```python
from build123d import *

# Parameters (mm, degrees)
F1_DEPTH = 63.5
F2_DEPTH = 25.4
F3_DEPTH = 7.9375
F5_R     = 6.35


with BuildPart() as f1:
    # F0 (on Front) → F1 (new body, symmetric)
    with BuildSketch(Plane.XZ):
        Polygon((12.7672983825, 16.0020012408), (-31.8172983825, 16.0020012408), (-31.8172983825, -16.0020012408), (31.8172983825, -16.0020012408), (31.8172983825, 16.0020012408), align=None)
    extrude(amount=F1_DEPTH, both=True)

    # F0 (on Front) → F2 (join, symmetric)
    with BuildSketch(Plane.XZ):
        with BuildLine():
            Line((12.7672983825, 20.5231987592), (12.7672983825, 16.0020012408))
            Line((12.7672983825, 16.0020012408), (31.8172983825, 16.0020012408))
            Line((31.8172983825, 16.0020012408), (31.8172983825, 20.5231987592))
            ThreePointArc((31.8172983825, 20.5231987592), (36.3344606658, 31.6144181421), (47.3152697086, 36.3937209427))
            Line((47.3152697086, 36.3937209427), (47.3152697086, 55.4461636158))
            ThreePointArc((47.3152697086, 55.4461636158), (22.8636521102, 45.0852416156), (12.7672983825, 20.5231987592))
        make_face()
        with BuildLine():
            ThreePointArc((47.6922983825, 55.4481987592), (47.5037812992, 55.4476899696), (47.3152697086, 55.4461636158))
            Line((47.3152697086, 55.4461636158), (47.3152697086, 36.3937209427))
            ThreePointArc((47.3152697086, 36.3937209427), (47.5037707507, 36.3970792656), (47.6922983825, 36.3981987592))
            Line((47.6922983825, 36.3981987592), (76.2672983825, 36.3981987592))
            Line((76.2672983825, 36.3981987592), (76.2672983825, 55.4481987592))
            Line((76.2672983825, 55.4481987592), (47.6922983825, 55.4481987592))
        make_face()
    extrude(amount=F2_DEPTH, both=True)

    # F0 (on Front) → F3 (join, symmetric)
    with BuildSketch(Plane.XZ):
        with BuildLine():
            add(Edge.make_bspline(
                [(47.3152697086, 55.447760652), (14.70907961, 55.3720610373), (-31.8172983825, 45.4738341579), (-31.8172983825, 16.0020012408)],
                knots=[0.3413515557, 0.3413515557, 0.3413515557, 0.3413515557, 88.7568503068, 88.7568503068, 88.7568503068, 88.7568503068], degree=3))
            Line((-31.8172983825, 16.0020012408), (12.7672983825, 16.0020012408))
            Line((12.7672983825, 16.0020012408), (12.7672983825, 20.5231987592))
            ThreePointArc((12.7672983825, 20.5231987592), (22.8636521102, 45.0852416156), (47.3152697086, 55.4461636158))
            Line((47.3152697086, 55.4461636158), (47.3152697086, 55.447760652))
        make_face()
    extrude(amount=F3_DEPTH, both=True)

    # F0 (on Front) → F4 (revolve)
    with BuildSketch(Plane.XZ):
        Polygon((98.1152697086, 60.1979987592), (76.2672983825, 60.1979987592), (76.2672983825, 55.4481987592), (76.2672983825, 36.3981987592), (76.2672983825, 31.6229987592), (98.1152697086, 31.6229987592), align=None)
    revolve(axis=Axis((76.2672983825, 0, 45.9104987592), (0, 0, -1)))

    # F5
    f5_edges = [f1.edges().sort_by_distance(p)[0] for p in [
        (31.817298, -63.5, 0),
        (-31.817298, -63.5, 0),
        (-31.817298, 63.5, 0),
        (31.817298, 63.5, 0),
        (0, -63.5, 16.002001),
        (0, -63.5, -16.002001),
        (31.817298, -44.45, 16.002001),
        (31.817298, 0, -16.002001),
        (-31.817298, 35.71875, 16.002001),
        (-31.817298, -35.71875, 16.002001),
        (-31.817298, 0, -16.002001),
        (0, 63.5, 16.002001),
        (0, 63.5, -16.002001),
        (31.817298, 44.45, 16.002001),
    ]]
    fillet(f5_edges, radius=F5_R)


solid = f1.part
```
Can you work these out from the model? Positions are in its coordinate system, mm. A direction names the side the tool comes from. Coordinates: 2 decimals unless noted, no trailing zeros. Loops run counter-clockwise (first coordinate to the right, second up) from the corner with the lowest first, then second, coordinate; pieces in that order, holes last. Notation, with made-up numbers: M 41,-22.75 L 73,-22.75 A26 cw 73,-0.75 Z; hole C 6,39 d4. An arc over 180 degrees is marked long. Put each result on its own line as item: value. Start each with the question number.
(1) Imagine slicing it at B-B on z = 0.5. List the corners of the cut face in (x, y) for me.
(2) Imagine slicing it at D-D on y = 12. List the corners of the cut face in (x, z) for me (3 decimals), and give its area (3 significant figures).
(3) Which directions (+Z, -Z, +X, -X, +Y, -Y) give clear straight access to the entire face, cutting with the end or side of a thin tool? Please do faces 1 (the face through (-2, 7.938, 33)), 2 (the face through (76.267, 24, 46)), 3 (the face through (76.267, -24, 46)), 4 (the face through (29.9, 41.5, 14.2)), 5 (the face through (-2, -7.938, 33)).
(4) Imagine slicing it at A-A on y = -40. List the corners of the cut face in (x, z) for me, and give its area (3 significant figures).
(5) I need wall thicknesses on probe 1 along Z at (x, y) = (-17.5, 20.5); probe 2 along X at (y, z) = (20.5, -8); probe 3 along Y at (x, z) = (35, 35). Which ranges of each line are inside material? Lowest first, please.
(6) Will these pins go through, and if not, where does the flat tip stop? pin 1 Ø8 at (y, z) = (17, 29.5) entering from +X; pin 2 Ø24.5 at (x, y) = (5.5, 22) entering from +Z; pin 3 Ø23 at (x, z) = (19, 31.5) entering from -Y.
(7) Imagine slicing it at C-C on x = 66. List the corners of the cut face in (y, z) for me.
(8) We'd pull the mould along X, two halves only. Please class faces 6 (the face through (30, -0.8, -14.1)), 7 (the face through (0, -1, -16.002)), 8 (the face through (-29.9, 32.9, 14.2)), 9 (the face through (52, 0, 36.398)): +X half, -X half, draft (parallel to the pull), parting line (faces both ways), or undercut.
Worked answers:
1. outline: M -31.82,-57.15 A6.35 ccw -25.47,-63.5 L 25.47,-63.5 A6.35 ccw 31.82,-57.15 L 31.82,57.15 A6.35 ccw 25.47,63.5 L -25.47,63.5 A6.35 ccw -31.82,57.15 Z
2. outline: M -31.817,-9.652 A6.35 ccw -25.467,-16.002 L 25.467,-16.002 A6.35 ccw 31.817,-9.652 L 31.817,20.523 A15.875 cw 47.692,36.398 L 58.01,36.398 L 58.01,31.623 L 94.525,31.623 L 94.525,60.198 L 58.01,60.198 L 58.01,55.448 L 47.692,55.448 A34.925 ccw 47.315,55.446 A34.925 ccw 12.767,20.523 L 12.767,16.002 L -25.467,16.002 A6.35 ccw -31.817,9.652 Z
2. area: 4,100 mm2
3. face 1: +Z, -X, +Y
3. face 2: +Z, -Z, +X, +Y
3. face 3: +Z, -Z, +X, -Y
3. face 4: +Z, +X, +Y
3. face 5: +Z, -X, -Y
4. outline: M -31.82,-9.65 A6.35 ccw -25.47,-16 L 25.47,-16 A6.35 ccw 31.82,-9.65 L 31.82,9.65 A6.35 ccw 25.47,16 L -25.47,16 A6.35 ccw -31.82,9.65 Z
4. area: 2,000 mm2
5. probe 1: z = -16 to 16
5. probe 2: x = -31.82 to 31.82
5. probe 3: y = -25.4 to 25.4
6. pin 1: stops at x = 93.36
6. pin 2: stops at z = 38.5
6. pin 3: stops at y = -25.4
7. outline: M -25.4,36.4 L -19.29,36.4 L -19.29,31.62 L 19.29,31.62 L 19.29,36.4 L 25.4,36.4 L 25.4,55.45 L 19.29,55.45 L 19.29,60.2 L -19.29,60.2 L -19.29,55.45 L -25.4,55.45 Z
8. face 6: +X half
8. face 7: draft
8. face 8: -X half
8. face 9: undercut
